from build123d import *

# Parameters (mm, degrees)
IZIM1_R                     = 167.5
IZIM1_R_2                   = 148
Y_KSEKLIK_EKSTR_ZYON2_DEPTH = 185.3
IZIM9_R                     = 3.4
KES_EKSTR_ZYON1_DEPTH       = 15
IZIM10_W                    = 5
IZIM10_H                    = 16.407796145


with BuildPart() as part:
    # Çizim1 → Yükseklik-Ekstrüzyon2 (new body)
    with BuildSketch(Plane.XY):
        Circle(IZIM1_R)
        Circle(IZIM1_R_2, mode=Mode.SUBTRACT)
    extrude(amount=Y_KSEKLIK_EKSTR_ZYON2_DEPTH)

    # Çizim9 → Kes-Ekstrüzyon1 (cut)
    with BuildSketch(Plane(origin=(0, 0, 0), x_dir=(-1, 0, 0), z_dir=(0, 0, -1))):
        with Locations((107.349895203, -112.5)):
            Circle(IZIM9_R)
        with Locations((-107.349895203, -112.5)):
            Circle(IZIM9_R)
        with Locations((-107.349895203, 112.5)):
            Circle(IZIM9_R)
        with Locations((107.349895203, 112.5)):
            Circle(IZIM9_R)
    kes_ekstr_zyon1 = extrude(amount=-KES_EKSTR_ZYON1_DEPTH, mode=Mode.SUBTRACT)

    # Çizim10 → Döndür1 (revolve)
    with BuildSketch(Plane(origin=(0, 0, 0), x_dir=(0, 0, -1), z_dir=(1, 0, 0)), mode=Mode.PRIVATE) as d_nd_r1_sk:
        with Locations((-32.5, 150.703898073)):
            Rectangle(IZIM10_W, IZIM10_H)
    revolve(d_nd_r1_sk.sketch.rotate(Axis((0, 0, 0), (0, 0, 1)), 90), axis=Axis((0, 0, 0), (0, 0, 1)))

    # Aynalama1: Kes-Ekstrüzyon1 across plane
    add(kes_ekstr_zyon1.mirror(Plane(origin=(0, 0, 92.65), x_dir=(1, 0, 0), z_dir=(0, 0, -1))), mode=Mode.SUBTRACT)


solid = part.part
Geometry: final body of the model. Coordinates: model frame, mm. A direction names the side the tool comes from. Round coordinates to 2 decimals unless told otherwise and drop trailing zeros. Loops run counter-clockwise (first coordinate to the right, second up) from the corner with the lowest first, then second, coordinate; pieces in that order, holes last.
Q1. Material intervals for L1, parallel to X at y = -2.5, z = 154.5; L2, parallel to Y at x = 0, z = 32; L3, parallel to X at y = -67.5, z = 50.5, sorted ascending.
Q2. Pin query (flat end, axial travel): P1, Ø8, axis at x = -107.35, y = -112.5, coming from the -Z side; P2, Ø6, axis at x = 24, z = 128.5, coming from the +Y side; P3, Ø1, axis at y = -107, z = 85, coming from the +X side; P4, Ø6, axis at x = -107.35, y = 112.5, coming from the -Z side. Return the tip coordinate at first contact, or that it passes through.
Q3. Access query for faces 4 (the cylindrical face through (-32.08, -144.48, 14.79)), 5 (the flat face through (12, -148, 185.3)), 6 (the cylindrical face through (-32.08, -144.48, 109.1)). Directions: +Z, -Z, +X, -X, +Y, -Y. A direction counts if a zero-diameter tool reaches every point of the face in a straight line with its end or side. Return the directions, or none.
Q4. Section C-C on z = 101.5. Return loops of the section in (x, y), plus the area to 3 significant figures.
Q5. Pull-direction query (X, two-part tool) for faces 1 (the flat face through (12, -148, 0)), 2 (the cylindrical face through (-132.922, -101.921, 91.353)), 3 (the flat face through (-77, -121, 35)); classes: released by +X, released by -X, zero draft, split by the parting line, or undercut.
Q6. Section A-A on y = 0. Return loops of the section in (x, z).
Evaluation:
1. L1: x = -167.48 to -147.98, 147.98 to 167.48
1. L2: y = -167.5 to -142.5, 142.5 to 167.5
1. L3: x = -153.3 to -131.71, 131.71 to 153.3
2. P1: stops at z = 0
2. P2: stops at y = 166.18
2. P3: stops at x = 129.28
2. P4: stops at z = 15
3. face 4: -Z
3. face 5: +Z, +X, -X, +Y, -Y
3. face 6: +Z
4. outline: circle Ø335 at (0, 0); hole circle Ø296 at (0, 0)
4. area: 19,300 mm2
5. face 1: zero draft
5. face 2: split by the parting line
5. face 3: undercut
6. outline: (-167.5, 0) - (-148, 0) - (-148, 30) - (-142.5, 30) - (-142.5, 35) - (-148, 35) - (-148, 185.3) - (-167.5, 185.3) - close; (142.5, 30) - (148, 30) - (148, 0) - (167.5, 0) - (167.5, 185.3) - (148, 185.3) - (148, 35) - (142.5, 35) - close
